Could you check a few things on this drawing? It's one solid part, dimensions in mm from its lowest x, y, z. A direction names the side the tool comes from. Give positions to 0.01 mm unless a question says otherwise; leave off trailing zeros. Write each loop counter-clockwise with the first axis right and the second up, starting at its lowest first coordinate (ties: lowest second). Pieces come first, ordered by that corner, then holes. Notation, with made-up numbers: (-40, 78) - (-19, 78) arc R27 cw to (-19, 95) - close; hole circle Ø3 at (-21, -4). An arc over 180 degrees is marked (long way). One line per item, written item: value. Start each with the question number.
1) Please list where these lines run through material, in increasing order: L1, parallel to Y at x = 11.5, z = 18; L2, parallel to Z at x = 3, y = 19.75; L3, parallel to Z at x = 6, y = 17.75. Write a range as [from, to].
2) On a 3-axis mill with a long thin cutter (end or side, diameter ignored), from which of +Z, -Z, +X, -X, +Y, -Y can I reach the whole of each face in a straight line? I mean the marked faces 1 and 2. Say none if no direction works.
3) I'm going to push flat-ended pins straight in: P1, Ø1.5, axis at x = 20.5, y = 12.5, coming from the +Z side; P2, Ø5, axis at x = 5, z = 7, coming from the +Y side; P3, Ø1.5, axis at x = 17.5, y = 19.5, coming from the -Z side; P4, Ø4, axis at x = 29, y = 16.5, coming from the +Z side. Where does each tip first touch, or does it pass through?
4) Imagine slicing it at C-C on z = 19. Write out the boundary of the cut face in (x, y).
5) Imagine slicing it at A-A on z = 7. Write out the boundary of the cut face in (x, y) (1 decimal), plus the area to 3 significant figures.
6) We'd pull the mould along Y, two halves only. Please class the marked faces 3, 4 and 5: +Y half, -Y half, draft (parallel to the pull), parting line (faces both ways), or undercut.
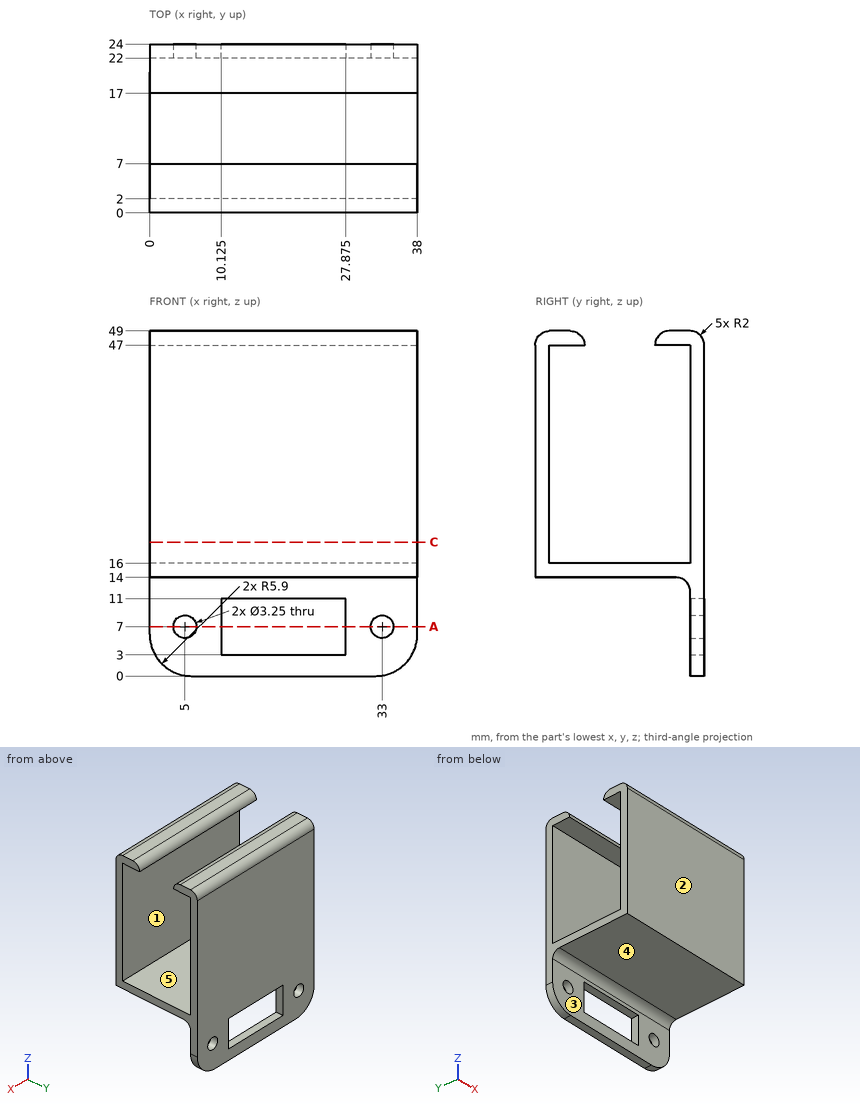
Numbers:
1. L1: [0, 2], [22, 24]
1. L2: [14, 16], [47, 49]
1. L3: [14, 16], [47, 48.56]
2. face 1: +X, -X
2. face 2: +Z, -Z, +X, -X, -Y
3. P1: z = 16
3. P2: y = 24
3. P3: z = 13.98
3. P4: z = 48.94
4. outline: (0, 0) - (38, 0) - (38, 2) - (0, 2) - close; (0, 22) - (38, 22) - (38, 24) - (0, 24) - close
5. outline: (0, 22) - (3.4, 22) - (3.4, 24) - (0, 24) - close; (6.6, 22) - (10.1, 22) - (10.1, 24) - (6.6, 24) - close; (27.9, 22) - (31.4, 22) - (31.4, 24) - (27.9, 24) - close; (34.6, 22) - (38, 22) - (38, 24) - (34.6, 24) - close
5. area: 27.5 mm^2
6. face 3: -Y half
6. face 4: draft
6. face 5: undercut
